Input: part model. Units: mm. Frame: model coordinates. Face numbers are marked on the shaded views. A direction names the side the tool comes from. Give positions to 0.01 mm unless a question says otherwise; leave off trailing zeros. Write each loop counter-clockwise with the first axis right and the second up, starting at its lowest first coordinate (ties: lowest second). Pieces come first, ordered by that corner, then holes. Notation, with made-up numbers: (79.5, 63.5) - (135.5, 63.5) arc R22 ccw to (135.5, 85.5) - close; hole circle Ø11 at (88.25, 14.25). An arc over 180 degrees is marked (long way). Answer as CSV lines item,"result".
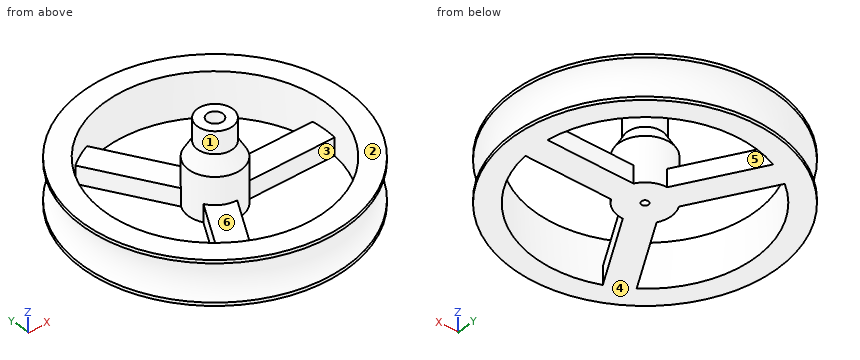
Autodesk Inventor part; units mm, degrees
ref_plane "YZ Plane" through (0, 0, 0) normal (1, 0, 0) x (0, 1, 0)
ref_plane "XZ Plane" through (0, 0, 0) normal (0, 1, 0) x (-1, 0, 0)
ref_plane "XY Plane" through (0, 0, 0) normal (0, 0, 1) x (1, 0, 0)
sketch "Sketch1" plane through (0, 0, 0) normal (0, 0, 1) x (1, 0, 0)
  circle A0 centre (0, 0) radius 15
  circle A1 centre (0, 0) radius 12.5
  dimension "d0" = 30
  dimension "d1" = 25
extrude "Extrusion1" add sketch "Sketch1" along normal blind 5
sketch "Sketch2" plane through (0, 0, 0) normal (0, 0, -1) x (-1, 0, 0)
  circle A0 centre (0, 0) radius 3
  dimension "d5" = 6
extrude "Extrusion2" add sketch "Sketch2" against normal blind 6.8
sketch "Sketch3" plane through (0, 0, 6.8) normal (0, 0, 1) x (1, 0, 0)
  circle A0 centre (0, 0) radius 2
  dimension "d8" = 4
extrude "Extrusion3" add sketch "Sketch3" along normal blind 2.5
chamfer "Chamfer1" distance 1 angle 60 1 edges at (3, 0, 6.8) measured on face at (-2.6182, -0.3989, 6.8)
sketch "Sketch4" plane through (0, 0, 9.3) normal (0, 0, 1) x (1, 0, 0)
  circle A0 centre (0, 0) radius 0.9
  dimension "d14" = 1.8
extrude "Extrusion4" cut sketch "Sketch4" against normal blind 4.8
sketch "Sketch5" plane through (0, 0, 0) normal (0, 0, -1) x (-1, 0, 0)
  line L0 (-2, 1.5) -> (-13, 1.5)
  line L1 (-13, 1.5) -> (-13, -1.5)
  line L2 (-13, -1.5) -> (-2, -1.5)
  line L3 (-2, -1.5) -> (-2, 1.5)
  circle A0 centre (0, 0) radius 0.9
  line L4 (0, 0) -> (-17.4633, 0) construction
  circle A1 centre (0, 0) radius 3
  circle A2 centre (0, 0) radius 12.5
  point P0 (-13, 0)
  point P1 (-12.4097, 1.5)
  point P2 (-12.4097, -1.5)
  point P3 (-2.5981, -1.5)
  point P4 (-2.5981, 1.5)
  dimension "d19" = 3
  dimension "d20" = 11
extrude "Extrusion6" add sketch "Sketch5" against normal blind 2 contours A1 L2 A2 L0 picked at (-9.3212, 0.1045)
pattern_circular "Circular Pattern2" count 3 over 360 about axis through (0, 0, -10) along (0, 0, 1) of "Extrusion6"
sketch "Sketch6" plane through (0, 0, 4.5) normal (0, 0, 1) x (1, 0, 0)
  circle A0 centre (0, 0) radius 2
  circle A1 centre (0, 0) radius 0.4
  dimension "d32" = 0.8
extrude "Extrusion7" cut sketch "Sketch6" against normal blind 5.3 contours A1
sketch "Sketch7" plane through (0, 0, 0) normal (0, 1, 0) x (-1, 0, 0)
  point P0 (0, 0)
sketch "Sketch8" plane through (0, 0, 0) normal (0, 1, 0) x (-1, 0, 0)
  line L0 (15, 0) -> (15, 5)
  circle A0 centre (16.3, 2.5) radius 2.5
  line L1 (0, 0) -> (0, 2)
  line L2 (0, 0) -> (0, 12.0754) construction
  point P0 (15, 2.5)
  point P1 (15, 4.6354)
  point P2 (15, 0.3646)
  dimension "d35" = 5
  dimension "d36" = 1.3
revolve "Revolution1" cut sketch "Sketch8" angle 360 about axis through (0, 0, 0) along (0, 0, 1)
properties part number "Koło"
Item 1: Cut plane B-B on z = 7.5. Return the cut outline in (x, y).
The answers:
outline,"circle Ø4 at (0, 0); hole circle Ø1.8 at (0, 0)"
Item 2: Mould query, pull axis X, two halves, no side actions, for the marked faces 1, 2 and 3. Classes: +X half, -X half, draft (parallel to the pull), parting line (faces both ways), or undercut.
The answers:
face 1,"parting line"
face 2,"draft"
face 3,"undercut"
Item 3: Cut plane C-C on z = 3.5. Return the cut outline in (x, y).
The answers:
outline,"circle Ø28.02 at (0, 0); circle Ø6 at (0, 0); hole circle Ø25 at (0, 0); hole circle Ø0.8 at (0, 0)"
Item 4: Cut plane A-A on y = 0. Count the separate pieces of the cut face and the enclosed holes in it, plus the area to 3 significant figures.
The answers:
separate pieces,"3"
enclosed holes,"0"
area,"73.6 mm²"
Item 5: Contact query for flat-ended pins moving along their axis: pin 1 (4 mm diameter, centred on x = -2, y = -8.5, fed in from +Z); pin 2 (3 mm diameter, centred on y = 5, z = 1.5, fed in from -X); pin 3 (2 mm diameter, centred on x = 7.5, z = 1, fed in from +Y). Output: stop coordinate, or through.
The answers:
pin 1,"z = 2"
pin 2,"x = -14.45"
pin 3,"y = 13.41"
Item 6: Ray query, line 1 (X direction, y = -2.75, z = 2.5); line 2 (Y direction, x = 0, z = 3.15); line 3 (Z direction, x = -6, y = -9). Return the intervals inside material, ascending. Write a range as from..to.
The answers:
line 1,"-13.52..-12.19, -1.2..1.2, 12.19..13.52"
line 2,"-13.89..-12.5, -3..-0.4, 0.4..3, 12.5..13.89"
line 3,"0..2"
Item 7: Reachability of the marked faces 4, 5 and 6 from +Z, -Z, +X, -X, +Y, -Y: full face, straight path, thin tool, end or side. Return the list, or none.
The answers:
face 4,"-Z, +X, -X, +Y, -Y"
face 5,"+Z, -Z"
face 6,"+Z"
